Design review of the part built by this model. Coordinates are the model's own, in mm. Round coordinates to 2 decimals unless told otherwise and drop trailing zeros. Loops run counter-clockwise (first coordinate to the right, second up) from the corner with the lowest first, then second, coordinate; pieces in that order, holes last. Notation, with made-up numbers: (61.25, 31.5) -> (76.25, 31.5) arc R32 cw to (76.25, 59.5) -> close; hole circle Ø2 at (87.25, -31). An arc over 180 degrees is marked (long way). Use a Markdown table: item, result. Add a question column.
from build123d import *

# Parameters (mm, degrees)
F1_DEPTH = 6
F2_SIZE  = 1


with BuildPart() as f1:
    # F0 (on Top) → F1 (new body)
    with BuildSketch(Plane.XY):
        with BuildLine():
            Line((-91, 7), (-94, 7))
            ThreePointArc((-94, 7), (-98.242641, 5.242641), (-100, 1))
            Line((-100, 1), (-100, -1))
            ThreePointArc((-100, -1), (-98.242641, -5.242641), (-94, -7))
            Line((-94, -7), (6.5, -7))
            ThreePointArc((6.5, -7), (10.742641, -5.242641), (12.5, -1))
            Line((12.5, -1), (12.5, 1))
            ThreePointArc((12.5, 1), (10.742641, 5.242641), (6.5, 7))
            Line((6.5, 7), (1, 7))
            ThreePointArc((1, 7), (0, 6), (-1, 7))
            Line((-1, 7), (-9, 7))
            ThreePointArc((-9, 7), (-10, 6), (-11, 7))
            Line((-11, 7), (-19, 7))
            ThreePointArc((-19, 7), (-20, 6), (-21, 7))
            Line((-21, 7), (-29, 7))
            ThreePointArc((-29, 7), (-30, 6), (-31, 7))
            Line((-31, 7), (-39, 7))
            ThreePointArc((-39, 7), (-40, 6), (-41, 7))
            Line((-41, 7), (-49, 7))
            ThreePointArc((-49, 7), (-50, 6), (-51, 7))
            Line((-51, 7), (-59, 7))
            ThreePointArc((-59, 7), (-60, 6), (-61, 7))
            Line((-61, 7), (-69, 7))
            ThreePointArc((-69, 7), (-70, 6), (-71, 7))
            Line((-71, 7), (-79, 7))
            ThreePointArc((-79, 7), (-80, 6), (-81, 7))
            Line((-81, 7), (-89, 7))
            ThreePointArc((-89, 7), (-90, 6), (-91, 7))
        make_face()
        with BuildLine():
            ThreePointArc((-69.49713, -4.5), (-69.996478, -4.025541), (-69.548145, -3.502609))
            Line((-69.548145, -3.502609), (-50.287825, -1.527192))
            ThreePointArc((-50.287825, -1.527192), (-50.022703, -1.513624), (-49.75758, -1.527161))
            Line((-49.75758, -1.527161), (-30.474618, -3.502603))
            ThreePointArc((-30.474618, -3.502603), (-30.026225, -4.025511), (-30.525574, -4.5))
            Line((-30.525574, -4.5), (-69.49713, -4.5))
        make_face(mode=Mode.SUBTRACT)
        with BuildLine():
            Line((-94, -1.119694), (-94, 1.119694))
            ThreePointArc((-94, 1.119694), (-93.142166, 3.049683), (-91.134725, 3.706126))
            Line((-91.134725, 3.706126), (-59.84956, 0.497391))
            ThreePointArc((-59.84956, 0.497391), (-59.400574, 0), (-59.84956, -0.497391))
            Line((-59.84956, -0.497391), (-91.134725, -3.706126))
            ThreePointArc((-91.134725, -3.706126), (-93.142166, -3.049683), (-94, -1.119694))
        make_face(mode=Mode.SUBTRACT)
        with BuildLine():
            ThreePointArc((-69.548145, 3.502609), (-69.996478, 4.025541), (-69.49713, 4.5))
            Line((-69.49713, 4.5), (-30.525574, 4.5))
            ThreePointArc((-30.525574, 4.5), (-30.026225, 4.025511), (-30.474618, 3.502603))
            Line((-30.474618, 3.502603), (-49.75758, 1.527161))
            ThreePointArc((-49.75758, 1.527161), (-50.022703, 1.513624), (-50.287825, 1.527192))
            Line((-50.287825, 1.527192), (-69.548145, 3.502609))
        make_face(mode=Mode.SUBTRACT)
        with BuildLine():
            ThreePointArc((-40.15044, -0.497391), (-40.599426, 0), (-40.15044, 0.497391))
            Line((-40.15044, 0.497391), (-8.865275, 3.706126))
            ThreePointArc((-8.865275, 3.706126), (-6.857834, 3.049683), (-6, 1.119694))
            Line((-6, 1.119694), (-6, -1.119694))
            ThreePointArc((-6, -1.119694), (-6.857834, -3.049683), (-8.865275, -3.706126))
            Line((-8.865275, -3.706126), (-40.15044, -0.497391))
        make_face(mode=Mode.SUBTRACT)
        with BuildLine():
            ThreePointArc((-1.785357, -1.75), (-2.5, 0), (-1.785357, 1.75))
            Line((-1.785357, 1.75), (1.785357, 1.75))
            ThreePointArc((1.785357, 1.75), (2.5, 0), (1.785357, -1.75))
            Line((1.785357, -1.75), (-1.785357, -1.75))
        make_face(mode=Mode.SUBTRACT)
    extrude(amount=F1_DEPTH)

    # F2
    f2_edges = [f1.edges().sort_by_distance(p)[0] for p in [
        (0, 1.75, 0),
        (-2.5, 0, 0),
        (2.5, 0, 0),
        (0, -1.75, 0),
    ]]
    chamfer(f2_edges, length=F2_SIZE)


solid = f1.part
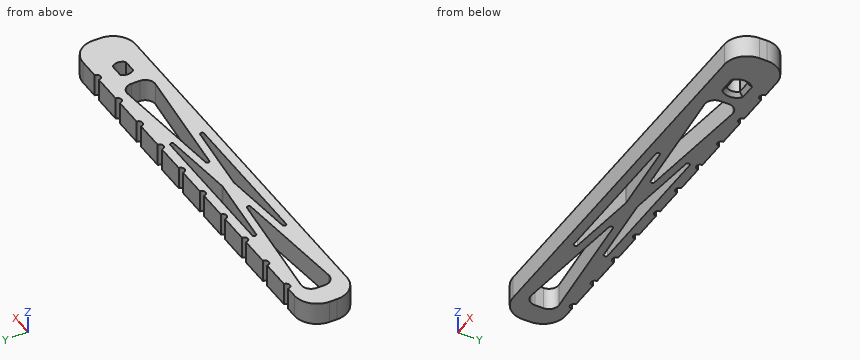
1. Consider section D-D on x = -86. State the section outline as (y, z) points, plus the area to 3 significant figures.
2. To check wall thickness, follow probe 1 along Y at (x, z) = (-53, 2); probe 2 along Y at (x, z) = (-50, 4); probe 3 along Y at (x, z) = (-72.5, 2.25). State the ranges of each line that lie inside material, in increasing order. Write a range as from..to.
3. Insertion check: P1, Ø2, axis at y = 5, z = 5, coming from the -X side. The pin has a flat end and moves straight along its axis. Give the tip position at first contact, or say it passes through.
4. Consider section A-A on x = -33.5. State the section outline as (y, z) points, plus the area to 3 significant figures.
5. Consider section B-B on x = 0. State the section outline as (y, z) points.
6. Consider section C-C on z = 3.5. Give the number of separate pieces and of enclosed holes in the cut face, plus the area to 3 significant figures.
Verdict:
| question | item | result |
|---|---|---|
| 1 | outline | (-7, 0) -> (-3.18, 0) -> (-3.18, 6) -> (-7, 6) -> close; (3.18, 0) -> (7, 0) -> (7, 6) -> (3.18, 6) -> close |
| 1 | area | 45.8 mm² |
| 2 | probe 1 | y = -7..-4.5, -1.81..1.81, 4.5..7 |
| 2 | probe 2 | y = -7..-4.5, -1.51..1.51, 4.5..6 |
| 2 | probe 3 | y = -7..-1.79, 1.79..7 |
| 3 | P1 | stops at x = -99.2 |
| 4 | outline | (-7, 0) -> (-4.5, 0) -> (-4.5, 6) -> (-7, 6) -> close; (-3.19, 0) -> (-1.18, 0) -> (-1.18, 6) -> (-3.19, 6) -> close; (1.18, 0) -> (3.19, 0) -> (3.19, 6) -> (1.18, 6) -> close; (4.5, 0) -> (7, 0) -> (7, 6) -> (4.5, 6) -> close |
| 4 | area | 54.2 mm² |
| 5 | outline | (-7, 0) -> (-2.75, 0) -> (-1.75, 1) -> (-1.75, 6) -> (-7, 6) -> close; (1.75, 1) -> (2.75, 0) -> (6, 0) -> (6, 6) -> (1.75, 6) -> close |
| 6 | separate pieces | 1 |
| 6 | enclosed holes | 5 |
| 6 | area | 1,050 mm² |
